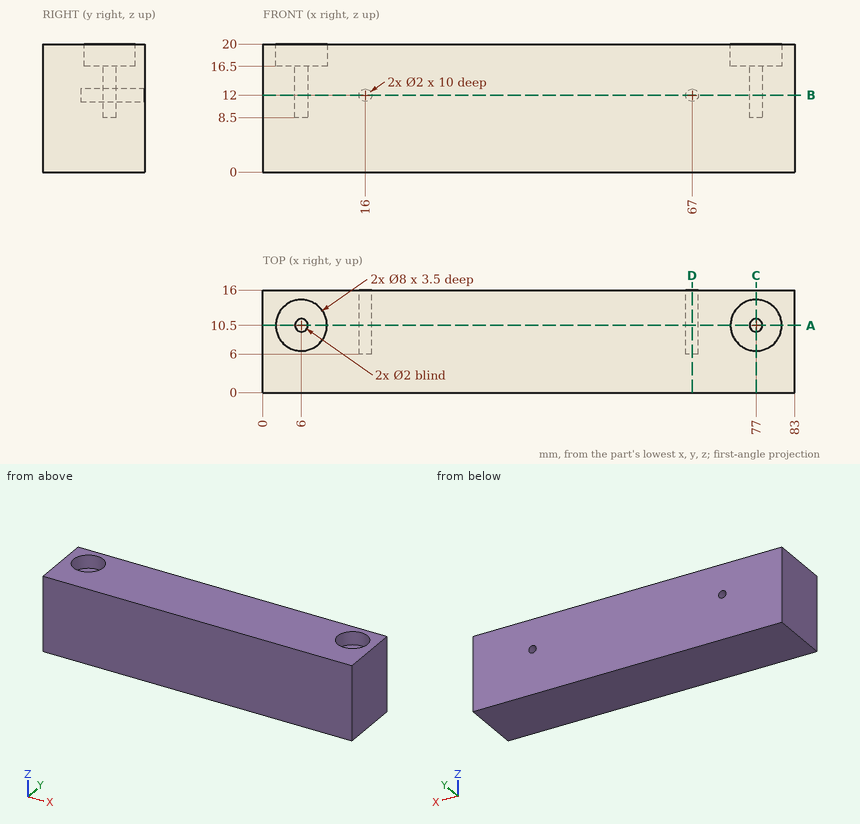
The figure shows three views and two pictorial views of one solid part (mm, origin at its lowest corner). Answer the questions. Give positions to 0.01 mm unless a question says otherwise; leave off trailing zeros. Write each loop counter-clockwise with the first axis right and the second up, starting at its lowest first coordinate (ties: lowest second). Pieces come first, ordered by that corner, then holes. Notation, with made-up numbers: (35.5, -27) - (46.5, -27) arc R34 cw to (46.5, 11) - close; hole circle Ø10 at (-20, -18.5). An arc over 180 degrees is marked (long way). Use CSV: the item, a comma, the result in double quotes. Start each with the question number.
Item 1: Consider line 1 (X direction, y = 13, z = 12); line 2 (Y direction, x = 6, z = 14); line 3 (Y direction, x = 6, z = 17.3). Determine where each line is inside the solid, lowest interval first.
Item 2: The part is cut by section C-C, the plane x = 77. Give the vertices of the cut face in (y, z).
Item 3: Flat-ended cylindrical pins translate along their axes: P1, Ø1.8, axis at x = 67, z = 12, coming from the +Y side; P2, Ø2, axis at x = 76.5, y = 10.5, coming from the +Z side; P3, Ø0.6, axis at x = 6, y = 11, coming from the +Z side. Find the tip coordinate at first contact, or state that the pin passes through.
Item 4: The part is cut by section B-B, the plane z = 12. Give the vertices of the cut face in (x, y).
Item 5: The part is cut by section A-A, the plane y = 10.5. Give the vertices of the cut face in (x, z), and give its area (3 significant figures).
Item 6: The part is cut by section D-D, the plane x = 67. Give the vertices of the cut face in (y, z), and give its area (3 significant figures).
Taken from the geometry:
1,line 1,"0 to 15, 17 to 66, 68 to 83"
1,line 2,"0 to 9.5, 11.5 to 16"
1,line 3,"0 to 6.5, 14.5 to 16"
2,outline,"(0, 0) - (16, 0) - (16, 20) - (14.5, 20) - (14.5, 16.5) - (11.5, 16.5) - (11.5, 8.5) - (9.5, 8.5) - (9.5, 16.5) - (6.5, 16.5) - (6.5, 20) - (0, 20) - close"
3,P1,"y = 6"
3,P2,"z = 16.5"
3,P3,"z = 8.5"
4,outline,"(0, 0) - (83, 0) - (83, 16) - (68, 16) - (68, 6) - (66, 6) - (66, 16) - (17, 16) - (17, 6) - (15, 6) - (15, 16) - (0, 16) - close; hole circle Ø2 at (6, 10.5); hole circle Ø2 at (77, 10.5)"
5,outline,"(0, 0) - (83, 0) - (83, 20) - (81, 20) - (81, 16.5) - (78, 16.5) - (78, 8.5) - (76, 8.5) - (76, 16.5) - (73, 16.5) - (73, 20) - (10, 20) - (10, 16.5) - (7, 16.5) - (7, 8.5) - (5, 8.5) - (5, 16.5) - (2, 16.5) - (2, 20) - (0, 20) - close; hole circle Ø2 at (16, 12); hole circle Ø2 at (67, 12)"
5,area,"1,570 mm2"
6,outline,"(0, 0) - (16, 0) - (16, 11) - (6, 11) - (6, 13) - (16, 13) - (16, 20) - (0, 20) - close"
6,area,"300 mm2"
